from build123d import *

# Parameters (mm, degrees)
F0_R     = 3.95
F1_DEPTH = 3.5
F2_R     = 6
F3_DEPTH = 2
F4_R     = 15
F5_DEPTH = 3
F6_SIZE  = 0.5
F7_SIZE  = 0.5
F8_SIZE2 = 0.35
F8_SIZE  = 0.35


with BuildPart() as f1:
    # F0 (on Front) → F1 (new body)
    with BuildSketch(Plane.XZ):
        Circle(F0_R)
    extrude(amount=F1_DEPTH)

    # F2 (on Front) → F3 (join)
    with BuildSketch(Plane.XZ):
        Circle(F2_R)
    extrude(amount=-F3_DEPTH)

    # F4 (on face) → F5 (join)
    with BuildSketch(Plane(origin=(0, 2, 0), x_dir=(-1, 0, 0), z_dir=(0, 1, 0))):
        Circle(F4_R)
    extrude(amount=F5_DEPTH)

    # F6
    f6_edges = [f1.edges().sort_by_distance(p)[0] for p in [
        (-3.95, -3.5, 0),
    ]]
    chamfer(f6_edges, length=F6_SIZE)

    # F7
    f7_edges = [f1.edges().sort_by_distance(p)[0] for p in [
        (-6, 0, 0),
        (15, 2, 0),
    ]]
    chamfer(f7_edges, length=F7_SIZE)

    # F8
    f8_edges = [f1.edges().sort_by_distance(p)[0] for p in [
        (15, 5, 0),
    ]]
    chamfer(f8_edges, length=F8_SIZE, length2=F8_SIZE2)


solid = f1.part
Input: part model. Units: mm. Frame: model coordinates. A direction names the side the tool comes from. Give positions to 0.01 mm unless a question says otherwise; leave off trailing zeros. Order: outer loops, then holes, each group sorted by start corner. A loop starts at its lowest first (then second) coordinate and runs counter-clockwise, first axis right, second up. Notation, with made-up numbers: (-3.75, 21) - (30.25, 21) arc R26 cw to (30.25, 38) - close; hole circle Ø11 at (85.25, -8). An arc over 180 degrees is marked (long way). Answer as a JSON object with one key per item and string values. Group by question number.
Q1. Set-up query: faces 1 (the face through (0, 5, 0)), 2 (the face through (-6.2, 2, 0.2)). Return all of +Z, -Z, +X, -X, +Y, -Y with unobstructed straight access to the full face (end or side cutting, diameter ignored); none if empty.
Q2. Cut plane C-C, the plane y = -0.75. Output: boundary loops of the cut face in (x, z).
Q3. Cut plane A-A, the plane x = 0. Output: boundary loops of the cut face in (y, z).
Q4. Cut plane B-B, the plane z = 0. Output: boundary loops of the cut face in (x, y), then the cut area to 3 significant figures.
Q5. Line query: probe 1 along X at (y, z) = (3.25, -0.25); probe 2 along Y at (x, z) = (-6.75, 5); probe 3 along X at (y, z) = (0.5, 0.25). Output: solid intervals per line, ascending.
Q6. First-contact query: pin 1 Ø1.5 at (x, y) = (-3, 0) entering from +Z; pin 2 Ø4 at (x, y) = (-5.5, 4) entering from -Z; pin 3 Ø2 at (y, z) = (4, -9) entering from +X. Flat tips, straight axial feed; report the tip coordinate or a pass-through.
Q7. Cut plane D-D, the plane y = 4.25. Output: boundary loops of the cut face in (x, z).
Results:
{
 "1": {"face 1": "+Z, -Z, +X, -X, +Y", "face 2": "-Y"},
 "2": {"outline": "circle Ø7.9 at (0, 0)"},
 "3": {"outline": "(-3.5, -3.45) - (-3, -3.95) - (0, -3.95) - (0, -5.5) - (0.5, -6) - (2, -6) - (2, -14.5) - (2.5, -15) - (4.65, -15) - (5, -14.65) - (5, 14.65) - (4.65, 15) - (2.5, 15) - (2, 14.5) - (2, 6) - (0.5, 6) - (0, 5.5) - (0, 3.95) - (-3, 3.95) - (-3.5, 3.45) - close"},
 "4": {"outline": "(-15, 2.5) - (-14.5, 2) - (-6, 2) - (-6, 0.5) - (-5.5, 0) - (-3.95, 0) - (-3.95, -3) - (-3.45, -3.5) - (3.45, -3.5) - (3.95, -3) - (3.95, 0) - (5.5, 0) - (6, 0.5) - (6, 2) - (14.5, 2) - (15, 2.5) - (15, 4.65) - (14.65, 5) - (-14.65, 5) - (-15, 4.65) - close", "area": "141 mm^2"},
 "5": {"probe 1": "-15 to 15", "probe 2": "2 to 5", "probe 3": "-5.99 to 5.99"},
 "6": {"pin 1": "z = 5.48", "pin 2": "z = -14.59", "pin 3": "x = 12.69"},
 "7": {"outline": "circle Ø30 at (0, 0)"}
}
